Source: CAD feature listing. Evaluate the final solid. Frame: model axes, mm. A direction names the side the tool comes from. Round coordinates to 2 decimals unless told otherwise and drop trailing zeros. Write each loop counter-clockwise with the first axis right and the second up, starting at its lowest first coordinate (ties: lowest second). Pieces come first, ordered by that corner, then holes. Notation, with made-up numbers: M 8,8.25 L 25,8.25 A22 ccw 25,36.25 Z; hole C 44,70.5 d10. An arc over 180 degrees is marked long. Answer in a Markdown table with one row per item. Add a question column.
Item 1: Cut plane A-A on z = -3.3. Return loops of the section in (x, y).
Item 2: Mould query, pull axis X, two halves, no side actions, for faces 4 (the face through (-411, 142, 0)), 5 (the face through (-406.266, 138.798, -1.974)), 6 (the face through (-411.34, 142.75, -1.97)). Classes: released by +X, released by -X, zero draft, split by the parting line, or undercut.
Item 3: Material intervals for probe 1 along Z at (x, y) = (-409.75, 136.5); probe 2 along Y at (x, z) = (-408.25, -1.1); probe 3 along X at (y, z) = (138.25, -2.7), sorted ascending.
Item 4: Set-up query: faces 1 (the face through (-405, 139, -0.3)), 2 (the face through (-411, 142, -4)), 3 (the face through (-405, 139, -3.7)). Return all of +Z, -Z, +X, -X, +Y, -Y with unobstructed straight access to the full face (end or side cutting, diameter ignored); none if empty.
Item 5: Contact query for a flat-ended pin moving along its axis: pin 1 (2.5 mm diameter, centred on x = -408.5, y = 139.5, fed in from -Z). Output: stop coordinate, or through.
from build123d import *

# Parameters (mm, degrees)
SKETCH_1_R          = 5
SKETCH_1_R_2        = 1.5
EXTRUDE_1_DEPTH     = 4
SKETCH_2_R          = 4
SKETCH_2_R_2        = 2.5
CUT_EXTRUDE_1_DEPTH = 0.3
CUT_EXTRUDE_START   = -3.7
SKETCH_2_2_R        = 4
SKETCH_2_2_R_2      = 2.5
CUT_EXTRUDE_3_DEPTH = 0.3
FILLET_1_R          = 0.15


with BuildPart() as part:
    # Эскиз1 → Бобышка-Вытянуть1 (new body)
    with BuildSketch(Plane.XY):
        with Locations((-407.651902974, 139.372619686)):
            Circle(SKETCH_1_R)
        with Locations((-407.651902974, 139.372619686)):
            Circle(SKETCH_1_R_2, mode=Mode.SUBTRACT)
    extrude(amount=-EXTRUDE_1_DEPTH)

    # Эскиз2 → Вырез-Вытянуть1 (cut)
    with BuildSketch(Plane.XY):
        with Locations((-407.651902974, 139.372619686)):
            Circle(SKETCH_2_R)
        with Locations((-407.651902974, 139.372619686)):
            Circle(SKETCH_2_R_2, mode=Mode.SUBTRACT)
    extrude(amount=-CUT_EXTRUDE_1_DEPTH, mode=Mode.SUBTRACT)

    # Эскиз2<2> → Вырез-Вытянуть3 (cut)
    with BuildSketch(Plane.XY.offset(CUT_EXTRUDE_START)):
        with Locations((-407.651902974, 139.372619686)):
            Circle(SKETCH_2_2_R)
        with Locations((-407.651902974, 139.372619686)):
            Circle(SKETCH_2_2_R_2, mode=Mode.SUBTRACT)
    extrude(amount=-CUT_EXTRUDE_3_DEPTH, mode=Mode.SUBTRACT)

    # Скругление1
    fillet_1_edges = [part.edges().sort_by_distance(p)[0] for p in [
        (-412.651902974, 139.372619686, 0),
        (-412.651902974, 139.372619686, -4),
        (-409.151902974, 139.372619686, -4),
        (-409.151902974, 139.372619686, 0),
    ]]
    fillet(fillet_1_edges, radius=FILLET_1_R)


solid = part.part
Results below:
| question | item | result |
|---|---|---|
| 1 | outline | C -407.65,139.37 d10; hole C -407.65,139.37 d3 |
| 2 | face 4 | zero draft |
| 2 | face 5 | undercut |
| 2 | face 6 | split by the parting line |
| 3 | probe 1 | -3.7 to -0.3 |
| 3 | probe 2 | 134.41 to 138, 140.75 to 144.34 |
| 3 | probe 3 | -412.52 to -408.65, -406.66 to -402.78 |
| 4 | face 1 | +Z |
| 4 | face 2 | -Z, +X, -X, +Y, -Y |
| 4 | face 3 | -Z |
| 5 | pin 1 | z = -4 |
